Geometry check sheet. Reference: the model listing, model coordinates, mm. Face numbers are marked on the shaded views. A direction names the side the tool comes from. Round coordinates to 2 decimals unless told otherwise and drop trailing zeros. Write each loop counter-clockwise with the first axis right and the second up, starting at its lowest first coordinate (ties: lowest second). Pieces come first, ordered by that corner, then holes. Notation, with made-up numbers: (82, 49) - (134, 49) arc R29 ccw to (134, 69) - close; hole circle Ø3 at (-39.5, 31). An arc over 180 degrees is marked (long way). One line per question, with ' | ' between items. Start each with the question number.
from build123d import *

# Parameters (mm, degrees)
F0_W      = 69.85
F0_H      = 38.1
F1_DEPTH  = 25.4
F2_W      = 44.45
F2_H      = 25.4
F3_DEPTH  = 25.4
F5_DEPTH  = 25.4
F7_DEPTH  = 25.4
F9_DEPTH  = 25.4
F10_R     = 6.349565
F11_DEPTH = 25.4


with BuildPart() as f1:
    # F0 (on Front) → F1 (new body)
    with BuildSketch(Plane.XZ):
        with Locations((34.925, 19.05)):
            Rectangle(F0_W, F0_H)
    extrude(amount=-F1_DEPTH)

    # F2 (on Front) → F3 (cut)
    with BuildSketch(Plane.XZ):
        with Locations((47.625, 25.4)):
            Rectangle(F2_W, F2_H)
    extrude(amount=-F3_DEPTH, mode=Mode.SUBTRACT)

    # F4 (on Top) → F5 (cut)
    with BuildSketch(Plane.XY):
        with BuildLine():
            ThreePointArc((63.5, 25.4), (68.174032, 19.799516), (69.85, 12.7))
            Line((69.85, 12.7), (69.85, 25.4))
            Line((69.85, 25.4), (63.5, 25.4))
        make_face()
        with BuildLine():
            ThreePointArc((69.85, 12.7), (68.174032, 5.600484), (63.5, 0))
            Line((63.5, 0), (69.85, 0))
            Line((69.85, 0), (69.85, 12.7))
        make_face()
    extrude(amount=F5_DEPTH, mode=Mode.SUBTRACT)

    # F6 (on Front) → F7 (cut)
    with BuildSketch(Plane.XZ):
        with BuildLine():
            ThreePointArc((0, 31.75), (5.663485, 36.425437), (12.814052, 38.1))
            Line((12.814052, 38.1), (0, 38.1))
            Line((0, 38.1), (0, 31.75))
        make_face()
        with BuildLine():
            ThreePointArc((12.814052, 38.1), (19.797928, 36.506847), (25.4, 32.042605))
            Line((25.4, 32.042605), (25.4, 38.1))
            Line((25.4, 38.1), (12.814052, 38.1))
        make_face()
    extrude(amount=-F7_DEPTH, mode=Mode.SUBTRACT)

    # F8 (on Top) → F9 (cut)
    with BuildSketch(Plane.XY):
        with BuildLine():
            Line((57.15, 19.05), (38.1, 19.05))
            ThreePointArc((38.1, 19.05), (31.75, 12.7), (38.1, 6.35))
            Line((38.1, 6.35), (57.15, 6.35))
            ThreePointArc((57.15, 6.35), (63.5, 12.7), (57.15, 19.05))
        make_face()
    extrude(amount=F9_DEPTH, mode=Mode.SUBTRACT)

    # F10 (on Front) → F11 (cut)
    with BuildSketch(Plane.XZ):
        with Locations((12.699565, 25.399565)):
            Circle(F10_R)
    extrude(amount=-F11_DEPTH, mode=Mode.SUBTRACT)


solid = f1.part
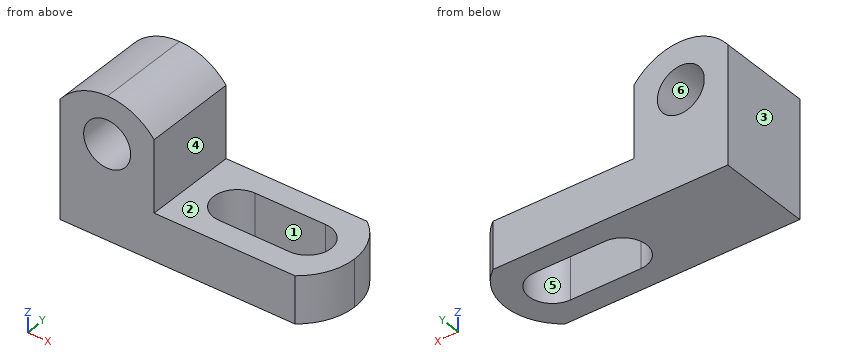
Q1. Section check A-A, the plane z = 3. Record the cut outline in (x, y) (3 decimals), then the cut area to 3 significant figures.
Q2. Section check B-B, the plane x = 47. Record the cut outline in (y, z), then the cut area to 3 significant figures.
Q3. Go/stop test with flat-tipped pins: P1, Ø9.5, axis at y = 10, z = 18, coming from the +X side; P2, Ø12, axis at x = 19, y = 7, coming from the +Z side. Record where each tip stops, or that it passes through.
Q4. Section check D-D, the plane z = 27.5. Record the cut outline in (x, y), then the cut area to 3 significant figures.
Q5. Section check C-C, the plane y = 13.75. Record the cut outline in (x, z), then the cut area to 3 significant figures.
Q6. Set-up check for the marked faces 4, 5 and 6: record each of +Z, -Z, +X, -X, +Y, -Y from which the full face is reachable in a straight line by a thin tool's end or side.
Q7. Thickness scan on line 1 (Y direction, x = 40.5, z = 8.5); line 2 (X direction, y = 23.75, z = 16). Record the ranges inside material, lowest first.
Q8. Draft check along X on the marked faces 1, 2 and 3. Enter one of: pulls with the +X half, pulls with the -X half, needs draft (parallel to the pull), parting line crosses it, or undercut.
Result sheet:
1) outline: (0, 0) - (63.5, 0) arc R15.875 ccw to (69.85, 12.7) arc R15.875 ccw to (63.5, 25.4) - (0, 25.4) - close; hole (38.1, 6.35) - (57.15, 6.35) arc R6.35 ccw to (57.15, 19.05) - (38.1, 19.05) arc R6.35 ccw to start | area: 1,360 mm²
2) outline: (0, 0) - (6.35, 0) - (6.35, 12.7) - (0, 12.7) - close; (19.05, 0) - (25.4, 0) - (25.4, 12.7) - (19.05, 12.7) - close | area: 161 mm²
3) P1: x = 25.4 | P2: z = 38.1
4) outline: (0, 0) - (6.71, 0) - (6.71, 25.4) - (0, 25.4) - close; (18.69, 0) - (25.4, 0) - (25.4, 25.4) - (18.69, 25.4) - close | area: 341 mm²
5) outline: (0, 0) - (31.84, 0) - (31.84, 12.7) - (25.4, 12.7) - (25.4, 32.04) arc R16.1 ccw to (12.81, 38.1) arc R16.1 ccw to (0, 31.75) - close; (63.41, 0) - (69.82, 0) - (69.82, 12.7) - (63.41, 12.7) - close; hole circle Ø12.7 at (12.7, 25.4) | area: 956 mm²
6) face 4: +Z, +X, +Y, -Y | face 5: +Z, -Z | face 6: +Y, -Y
7) line 1: 0 to 6.35, 19.05 to 25.4 | line 2: 0 to 25.4
8) face 1: undercut | face 2: needs draft | face 3: pulls with the -X half
